The figure shows three views and two pictorial views of one solid part (mm, origin at its lowest corner). Answer the questions. A direction names the side the tool comes from. Coordinates: 2 decimals unless noted, no trailing zeros. Loops run counter-clockwise (first coordinate to the right, second up) from the corner with the lowest first, then second, coordinate; pieces in that order, holes last.
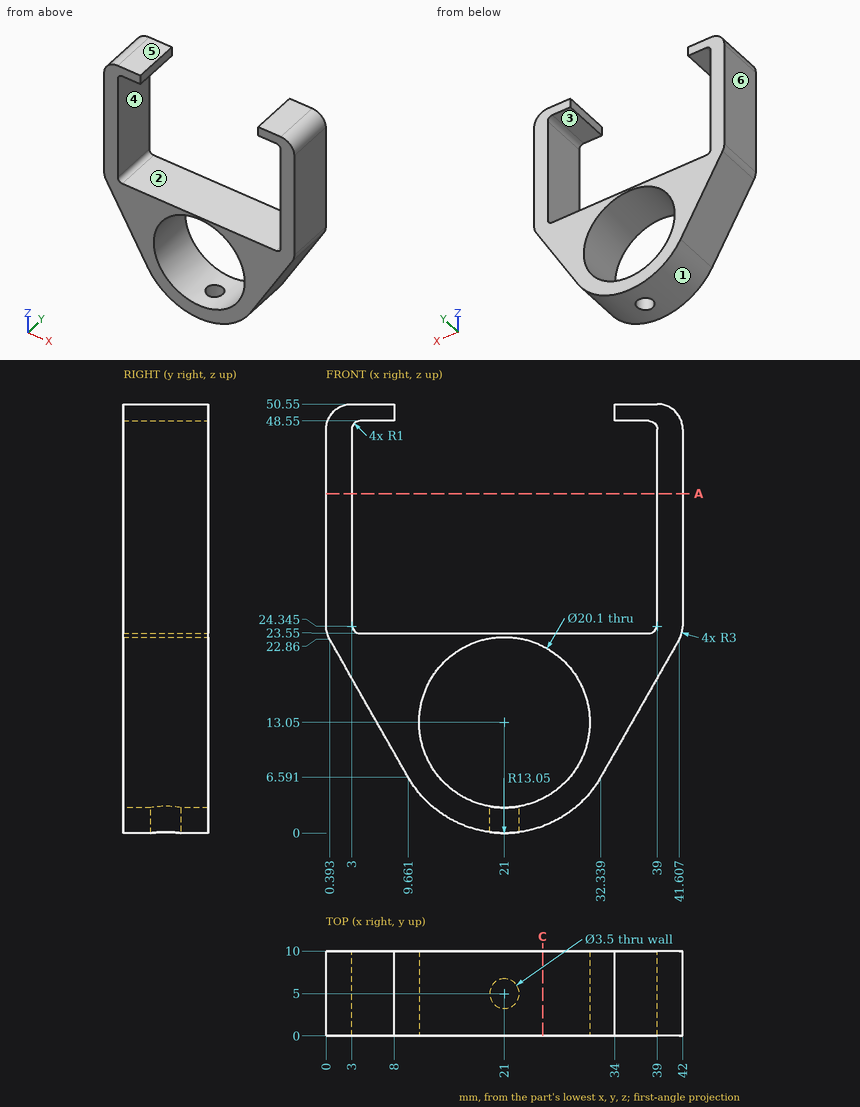
Q1. Determine the mould class of the marked faces 3, 4, 5 and 6 for opening direction Z: +Z half, -Z half, draft (parallel to the pull), parting line (faces both ways), or undercut.
Findings below:
face 3: undercut
face 4: undercut
face 5: +Z half
face 6: draft
Q2. Which of the six approach directions +Z, -Z, +X, -X, +Y, -Y give full straight-line access (tool end or side, diameter ignored) to the marked faces 1 and 2?
Findings below:
face 1: -Z, +Y, -Y
face 2: +Y, -Y
Q3. Flat-ended cylindrical pins translate along their axes: pin 1 Ø3 at (x, y) = (35.5, 6) entering from -Z (1 decimal); pin 2 Ø4.5 at (x, y) = (6, 6.5) entering from -Z (1 decimal); pin 3 Ø5.5 at (x, y) = (21, 5) entering from +Z; pin 4 Ø5 at (y, z) = (6.5, 36) entering from -X. Find the tip coordinate at first contact, or state that the pin passes through.
Findings below:
pin 1: stops at z = 9.5
pin 2: stops at z = 9.1
pin 3: stops at z = 23.55
pin 4: stops at x = 0
Q4. A cutting plane is placed at A-A (z = 40). Give the vertices of the cut face in (x, y), then the cut area to 3 significant figures.
Findings below:
outline: (0, 0) - (3, 0) - (3, 10) - (0, 10) - close; (39, 0) - (42, 0) - (42, 10) - (39, 10) - close
area: 60.0 mm2
Q5. A cutting plane is placed at C-C (x = 25.5). Give the vertices of the cut face in (y, z).
Findings below:
outline: (0, 0.8) - (10, 0.8) - (10, 4.06) - (0, 4.06) - close; (0, 22.04) - (10, 22.04) - (10, 23.55) - (0, 23.55) - close
Q6. Straight lines are drawn through the part: probe 1 along Y at (x, z) = (21, 1.3); probe 2 along X at (y, z) = (5, 30.5); probe 3 along X at (y, z) = (3, 7) (1 decimal). For each, find the intervals that lie inside material, in ascending order.
Findings below:
probe 1: y = 0 to 3.25, 6.75 to 10
probe 2: x = 0 to 3, 39 to 42
probe 3: x = 9.4 to 13, 29 to 32.6
